Can you work these out from the drawing? Everything is in mm from the part's minimum corner. A direction names the side the tool comes from. Round coordinates to 2 decimals unless told otherwise and drop trailing zeros. Write each loop counter-clockwise with the first axis right and the second up, starting at its lowest first coordinate (ties: lowest second). Pieces come first, ordered by that corner, then holes. Notation, with made-up numbers: (38.5, 61) - (80.5, 61) arc R28 ccw to (80.5, 83) - close; hole circle Ø5 at (-14.75, 3.5). An arc over 180 degrees is marked (long way). Write each question's results on one line, items separated by ' | '. Start each with the question number.
(1) Imagine slicing it at B-B on z = 10. Write out the boundary of the cut face in (x, y), then the cut area to 3 significant figures.
(2) For P1, Ø3.5, axis at x = 17.5, y = 17.5, coming from the +Z side; P2, Ø6, axis at x = 15.5, y = 19.5, coming from the -Z side; P3, Ø6, axis at y = 8, z = 17.5, coming from the +X side, each with a flat end and sliding along its axis, tell me the tip position at first contact or that it passes through.
(3) Imagine slicing it at D-D on z = 7.5. Write out the boundary of the cut face in (x, y).
(4) Please list where these lines run through material, in increasing order: line 1 (Y direction, x = 10, z = 16.75); line 2 (Y direction, x = 8, z = 13.5); line 3 (X direction, y = 17, z = 7). Write a range as [from, to].
(5) On a 3-axis mill with a long thin cutter (end or side, diameter ignored), from which of +Z, -Z, +X, -X, +Y, -Y can I reach the whole of each face in a straight line? I mean the marked faces 4, 5, 6, 7 and 8. Say none if no direction works.
(6) Thinking about a two-plate mould opening in X: for the marked faces 1, 2 and 3, which applies, +X half, -X half, draft (parallel to the pull), parting line (faces both ways), or undercut?
(7) Imagine slicing it at A-A on y = 13.25. Write out the boundary of the cut face in (x, z), then the cut area to 3 significant figures.
(8) Imagine slicing it at C-C on x = 10.5. Write out the boundary of the cut face in (y, z).
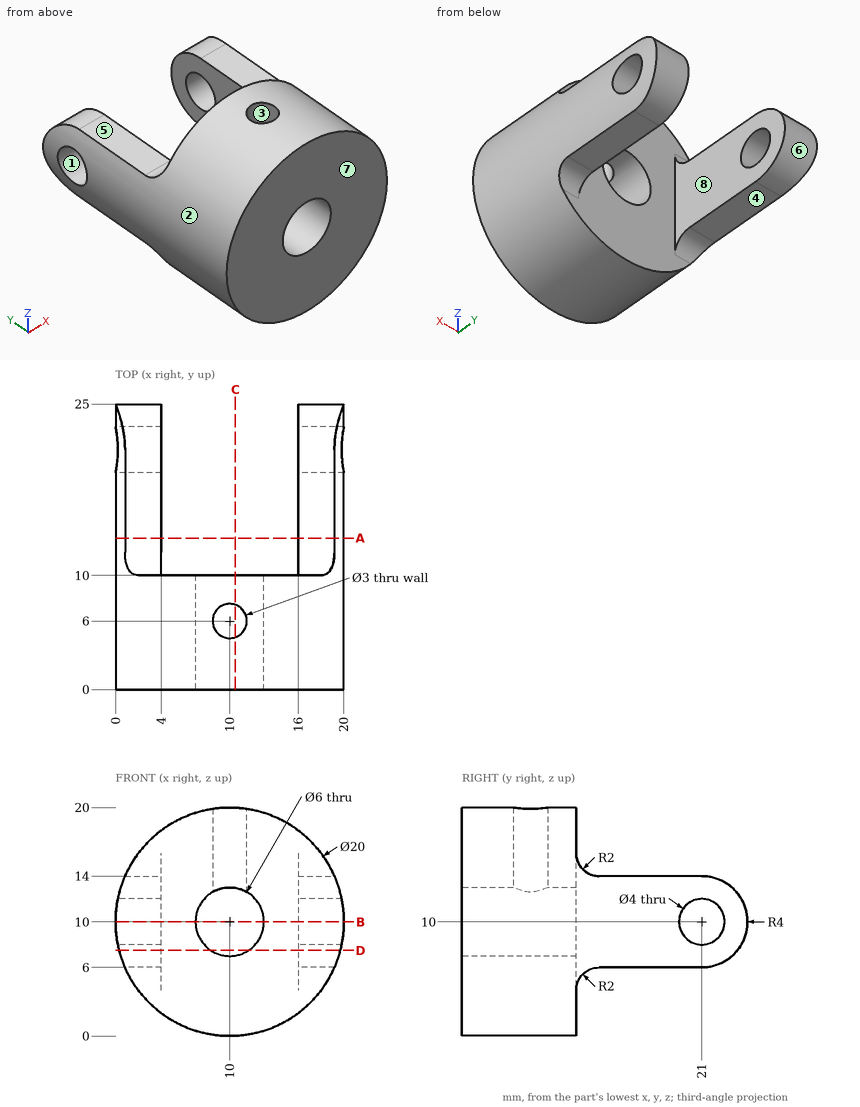
Response:
1) outline: (0, 0) - (7, 0) - (7, 10) - (4, 10) - (4, 19) - (0, 19) - close; (0, 23) - (4, 23) - (4, 25) - (0, 25) - close; (13, 0) - (20, 0) - (20, 19) - (16, 19) - (16, 10) - (13, 10) - close; (16, 23) - (20, 23) - (20, 25) - (16, 25) - close | area: 228 mm²
2) P1: z = 14 | P2: z = 6 | P3: x = 18.93
3) outline: (0.32, 0) - (8.34, 0) - (8.34, 10) - (4, 10) - (4, 24.12) - (0.32, 24.12) - close; (11.66, 0) - (19.68, 0) - (19.68, 24.12) - (16, 24.12) - (16, 10) - (11.66, 10) - close
4) line 1: [0, 4.5], [7.5, 10] | line 2: [0, 10] | line 3: [0.46, 4], [16, 19.54]
5) face 4: -Z, +X, -X, +Y | face 5: +Z, +X, -X, +Y | face 6: +X, -X, +Y | face 7: +Z, -Z, +X, -X, -Y | face 8: +Z, -Z, +Y
6) face 1: draft | face 2: parting line | face 3: undercut
7) outline: (0.83, 6) - (4, 6) - (4, 14) - (0.83, 14) arc R10 ccw to start; (16, 6) - (19.17, 6) arc R10 ccw to (19.17, 14) - (16, 14) - close | area: 59.6 mm²
8) outline: (0, 0.01) - (10, 0.01) - (10, 7.04) - (0, 7.04) - close; (0, 12.96) - (4.59, 12.96) - (4.59, 19.99) - (0, 19.99) - close; (7.41, 12.96) - (10, 12.96) - (10, 19.99) - (7.41, 19.99) - close
